```python
from build123d import *

# Parameters (mm, degrees)
F0_R     = 4
F0_W     = 9
F0_H     = 15
F0_W_2   = 2
F0_H_2   = 4
F0_W_3   = 9.720032
F0_H_3   = 15.864611
F0_W_4   = 6
F0_H_4   = 20
F1_DEPTH = 9


with BuildPart() as f1:
    # F0 (on Top) → F1 (new body)
    with BuildSketch(Plane.XY):
        Polygon((-16, 140), (-40, 140), (-141.243557, -35.358984), (-123.243557, -66.535898), (-112.851252, -60.535898), (-102.851252, -77.856406), (-113.243557, -83.856406), (-101.243557, -104.641016), (101.243557, -104.641016), (119.243557, -73.464102), (108.851252, -67.464102), (118.851252, -50.143594), (129.243557, -56.143594), (141.243557, -35.358984), (40, 140), (4, 140), (4, 128), (-16, 128), align=None)
        with Locations((-95.851252, -89.980762)):
            Circle(F0_R, mode=Mode.SUBTRACT)
        Polygon((-76.242984, -77.505223), (-72.778882, -75.505223), (-71.778882, -77.237274), (-75.242984, -79.237274), align=None, mode=Mode.SUBTRACT)
        Polygon((-100.173051, -59.151278), (-86.433895, -51.218972), (-81.573879, -59.636768), (-95.313035, -67.569073), align=None, mode=Mode.SUBTRACT)
        with Locations((-125.851252, -38.019238)):
            Circle(F0_R, mode=Mode.SUBTRACT)
        Polygon((-119.351252, -49.277568), (-122.351252, -44.081416), (-105.030744, -34.081416), (-102.030744, -39.277568), align=None, mode=Mode.SUBTRACT)
        Polygon((-99.242984, -37.668054), (-100.242984, -35.936003), (-96.778882, -33.936003), (-95.778882, -35.668054), align=None, mode=Mode.SUBTRACT)
        with Locations((-49.5, -23.646934)):
            Rectangle(F0_W, F0_H, mode=Mode.SUBTRACT)
        with Locations((95.851252, -89.980762)):
            Circle(F0_R, mode=Mode.SUBTRACT)
        Polygon((102.351252, -78.722432), (99.351252, -83.918584), (82.030744, -73.918584), (85.030744, -68.722432), align=None, mode=Mode.SUBTRACT)
        Polygon((82.242984, -67.112918), (81.242984, -68.844969), (77.778882, -66.844969), (78.778882, -65.112918), align=None, mode=Mode.SUBTRACT)
        Polygon((101.313035, -57.176768), (87.573879, -49.244463), (92.433895, -40.826667), (106.173051, -48.758973), align=None, mode=Mode.SUBTRACT)
        with Locations((49.5, -23.646934)):
            Rectangle(F0_W, F0_H, mode=Mode.SUBTRACT)
        Polygon((105.242984, -27.275749), (101.778882, -25.275749), (102.778882, -23.543698), (106.242984, -25.543698), align=None, mode=Mode.SUBTRACT)
        with Locations((125.851252, -38.019238)):
            Circle(F0_R, mode=Mode.SUBTRACT)
        with Locations((-49.5, 36.353066)):
            Rectangle(F0_W, F0_H, mode=Mode.SUBTRACT)
        with Locations((-30, 102.780972)):
            Rectangle(F0_W_2, F0_H_2, mode=Mode.SUBTRACT)
        with Locations((-6, 108.39574)):
            Rectangle(F0_W_3, F0_H_3, mode=Mode.SUBTRACT)
        with Locations((-30, 128)):
            Circle(F0_R, mode=Mode.SUBTRACT)
        with Locations((49.5, 36.353066)):
            Rectangle(F0_W, F0_H, mode=Mode.SUBTRACT)
        with BuildLine():
            Line((-7.5, 80.75011), (7.5, 80.75011))
            ThreePointArc((7.5, 80.75011), (11.035534, 79.285643), (12.5, 75.75011))
            Line((12.5, 75.75011), (12.5, 50.75011))
            ThreePointArc((12.5, 50.75011), (11.035534, 47.214576), (7.5, 45.75011))
            Line((7.5, 45.75011), (-7.5, 45.75011))
            ThreePointArc((-7.5, 45.75011), (-11.035534, 47.214576), (-12.5, 50.75011))
            Line((-12.5, 50.75011), (-12.5, 75.75011))
            ThreePointArc((-12.5, 75.75011), (-11.035534, 79.285643), (-7.5, 80.75011))
        make_face(mode=Mode.SUBTRACT)
        with Locations((18, 102.780972)):
            Rectangle(F0_W_2, F0_H_2, mode=Mode.SUBTRACT)
        with Locations((20, 118)):
            Rectangle(F0_W_4, F0_H_4, mode=Mode.SUBTRACT)
        with Locations((30, 128)):
            Circle(F0_R, mode=Mode.SUBTRACT)
    extrude(amount=F1_DEPTH)


solid = f1.part
```
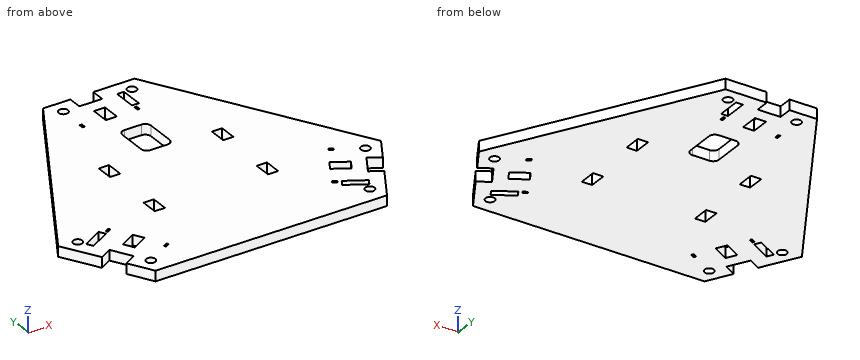
Source: CAD feature listing. Evaluate the final solid. Frame: model axes, mm. Give positions to 0.01 mm unless a question says otherwise; leave off trailing zeros. Write each loop counter-clockwise with the first axis right and the second up, starting at its lowest first coordinate (ties: lowest second). Pieces come first, ordered by that corner, then holes. Notation, with made-up numbers: (41, 62) - (75, 62) arc R29 ccw to (75, 97) - close; hole circle Ø3 at (-37, -28). An arc over 180 degrees is marked (long way). One line per item, written item: value. Start each with the question number.
Q1. Section query D-D, the plane y = 20.5. Return the cut outline in (x, z), then the cut area to 3 significant figures.
Q2. Section query C-C, the plane z = 2.5. Count the separate pieces of the cut face and the enclosed holes in it, then the cut area to 3 significant figures.
Q3. Section query A-A, the plane x = 30. Return the cut outline in (y, z), then the cut area to 3 significant figures.
Q4. First-contact query: pin 1 Ø4.5 at (y, z) = (134, 5.5) entering from -X; pin 2 Ø5 at (y, z) = (64, 1) entering from -X; pin 3 Ø1.2 at (y, z) = (103.5, 4.5) entering from +X. Flat tips, straight axial feed; report the tip coordinate or a pass-through.
Q5. Material intervals for probe 1 along Y at (x, z) = (-30, 3); probe 2 along X at (y, z) = (29, 4.25); probe 3 along X at (y, z) = (-50.5, 2), sorted ascending. Write a range as from..to.
Q6. Section query B-B, the plane y = 63. Return the cut outline in (x, z), then the cut area to 3 significant figures.
Answer:
1. outline: (-108.99, 0) - (108.99, 0) - (108.99, 9) - (-108.99, 9) - close
1. area: 1,960 mm2
2. separate pieces: 1
2. enclosed holes: 23
2. area: 45,300 mm2
3. outline: (-104.64, 0) - (124, 0) - (124, 9) - (-104.64, 9) - close; (132, 0) - (140, 0) - (140, 9) - (132, 9) - close
3. area: 2,130 mm2
4. pin 1: stops at x = -44.76
4. pin 2: stops at x = -85.32
4. pin 3: stops at x = 61.42
5. probe 1: y = -104.64..100.78, 104.78..124, 132..140
5. probe 2: x = -104.09..-54, -45..45, 54..104.09
5. probe 3: x = -132.5..89.75, 105.17..118.65, 119.47..132.5
6. outline: (-84.46, 0) - (-12.5, 0) - (-12.5, 9) - (-84.46, 9) - close; (12.5, 0) - (84.46, 0) - (84.46, 9) - (12.5, 9) - close
6. area: 1,300 mm2
